Can you work these out from the model? Positions are in its coordinate system, mm. A direction names the side the tool comes from. Round coordinates to 2 decimals unless told otherwise and drop trailing zeros. Loops run counter-clockwise (first coordinate to the right, second up) from the corner with the lowest first, then second, coordinate; pieces in that order, holes last. Notation, with made-up numbers: M -39.5,31 L 2.5,31 A27 ccw 2.5,50 Z; hole C -14.5,5 d9. An arc over 180 degrees is marked long. Return JSON: item names as keys, results as strings.
```python
from build123d import *

# Parameters (mm, degrees)
SKETCH2_W           = 150
SKETCH2_H           = 150
BOSS_EXTRUDE1_DEPTH = 1035
SKETCH3_W           = 100
SKETCH3_H           = 50
CUT_EXTRUDE3_DEPTH  = 935
SKETCH4_W           = 150
SKETCH4_H           = 30
CUT_EXTRUDE4_DEPTH  = 935
FILLET1_R           = 10
SKETCH5_R           = 45
BOSS_EXTRUDE2_DEPTH = 20
BOSS_EXTRUDE3_START = -45
SKETCH6_W           = 100
SKETCH6_H           = 75
BOSS_EXTRUDE3_DEPTH = 90
SKETCH7_W           = 60
SKETCH7_H           = 110
CUT_EXTRUDE5_DEPTH  = 90


with BuildPart() as part:
    # Sketch2 → Boss-Extrude1 (new body)
    with BuildSketch(Plane(origin=(0, 0, 0), x_dir=(1, 0, 0), z_dir=(0, 1, 0))):
        Rectangle(SKETCH2_W, SKETCH2_H)
    extrude(amount=BOSS_EXTRUDE1_DEPTH)

    # Sketch3 → Cut-Extrude3 (cut)
    with BuildSketch(Plane(origin=(0, 1035, 0), x_dir=(-1, 0, 0), z_dir=(0, 1, 0))):
        with Locations((0, -50)):
            Rectangle(SKETCH3_W, SKETCH3_H)
        with Locations((0, 50)):
            Rectangle(SKETCH3_W, SKETCH3_H)
    extrude(amount=-CUT_EXTRUDE3_DEPTH, mode=Mode.SUBTRACT)

    # Sketch4 → Cut-Extrude4 (cut)
    with BuildSketch(Plane(origin=(0, 1035, 0), x_dir=(-1, 0, 0), z_dir=(0, 1, 0))):
        with Locations((0, -60)):
            Rectangle(SKETCH4_W, SKETCH4_H)
        with Locations((0, 60)):
            Rectangle(SKETCH4_W, SKETCH4_H)
    extrude(amount=-CUT_EXTRUDE4_DEPTH, mode=Mode.SUBTRACT)

    # Fillet1
    fillet1_edges = [part.edges().sort_by_distance(p)[0] for p in [
        (0, 1035, -25),
        (50, 1035, -35),
        (0, 1035, 25),
        (-50, 1035, 35),
        (-50, 1035, -35),
        (-75, 1035, 0),
        (-62.5, 1035, -45),
        (62.5, 1035, -45),
        (50, 1035, 35),
        (75, 1035, 0),
        (62.5, 1035, 45),
        (-62.5, 1035, 45),
    ]]
    fillet(fillet1_edges, radius=FILLET1_R)

    # Sketch5 → Boss-Extrude2 (add)
    with BuildSketch(Plane(origin=(0, 1035, 0), x_dir=(-1, 0, 0), z_dir=(0, 1, 0))):
        with Locations(Location((0, 0, 0), (0, 0, 199.471220634))):
            Circle(SKETCH5_R)
    extrude(amount=BOSS_EXTRUDE2_DEPTH)

    # Sketch6 → Boss-Extrude3 (add)
    with BuildSketch(Plane.XY.offset(BOSS_EXTRUDE3_START)):
        with Locations((0, 1092.5)):
            Rectangle(SKETCH6_W, SKETCH6_H)
    extrude(amount=BOSS_EXTRUDE3_DEPTH)

    # Sketch7 → Cut-Extrude5 (cut)
    with BuildSketch(Plane.XY.offset(45)):
        with Locations((0, 1130)):
            Rectangle(SKETCH7_W, SKETCH7_H)
    extrude(amount=-CUT_EXTRUDE5_DEPTH, mode=Mode.SUBTRACT)


solid = part.part
```
Q1. I'm going to push flat-ended pins straight in: pin 1 Ø8 at (x, z) = (-2.5, 36) entering from +Y; pin 2 Ø25 at (x, z) = (-51.5, 16.5) entering from +Y; pin 3 Ø3 at (x, y) = (18, 145) entering from +Z; pin 4 Ø20 at (x, y) = (57, 643.5) entering from +Z. Where does each tip first touch, or does it pass through?
Results:
{"pin 1": "stops at y = 1075", "pin 2": "stops at y = 1130", "pin 3": "stops at z = 25", "pin 4": "stops at z = 45"}
Q2. Suppose I cut it at A-A, the plane y = 617.5. Please give me the cut outline in (x, z).
Results:
{"outline": "M -75,-45 L -50,-45 L -50,-25 L 50,-25 L 50,-45 L 75,-45 L 75,45 L 50,45 L 50,25 L -50,25 L -50,45 L -75,45 Z"}
Q3. If I drill on line 1 along Y through (x, z) = (9, 36); line 2 along X through (y, z) = (154.5, -35); line 3 along Z through (x, y) = (8.5, 235.5), over which ranges is the centre line in solid material (lowest first)?
Results:
{"line 1": "y = 0 to 100, 1035 to 1075", "line 2": "x = -75 to -50, 50 to 75", "line 3": "z = -25 to 25"}
Q4. Suppose I cut it at B-B, the plane z = 0. Please give me the cut outline in (x, y), plus the area to 3 significant figures.
Results:
{"outline": "M -75,0 L 75,0 L 75,1025 A10 ccw 65,1035 L 45,1035 L 45,1055 L 50,1055 L 50,1130 L 30,1130 L 30,1075 L -30,1075 L -30,1130 L -50,1130 L -50,1055 L -45,1055 L -45,1035 L -65,1035 A10 ccw -75,1025 Z", "area": "161,000 mm2"}
Q5. Suppose I cut it at C-C, the plane x = 13.5. Please give me the cut outline in (y, z).
Results:
{"outline": "M 0,-75 L 100,-75 L 100,-25 L 1025,-25 A10 ccw 1035,-15 L 1035,-42.93 L 1055,-42.93 L 1055,-45 L 1075,-45 L 1075,45 L 1055,45 L 1055,42.93 L 1035,42.93 L 1035,15 A10 ccw 1025,25 L 100,25 L 100,75 L 0,75 Z"}
Q6. On a 3-axis mill with a long thin cutter (end or side, diameter ignored), from which of +Z, -Z, +X, -X, +Y, -Y can I reach the whole of each face in a straight line? I mean faces 1 (the cylindrical face through (32.9, 1044.9, 30.7)), 2 (the flat face through (1, 100, -50)), 3 (the flat face through (50, 1092, -1)), 4 (the flat face through (45.3, 1055, -0.2)). Say none if no direction works.
Results:
{"face 1": "none", "face 2": "-Z", "face 3": "+Z, -Z, +X, +Y", "face 4": "+X"}
